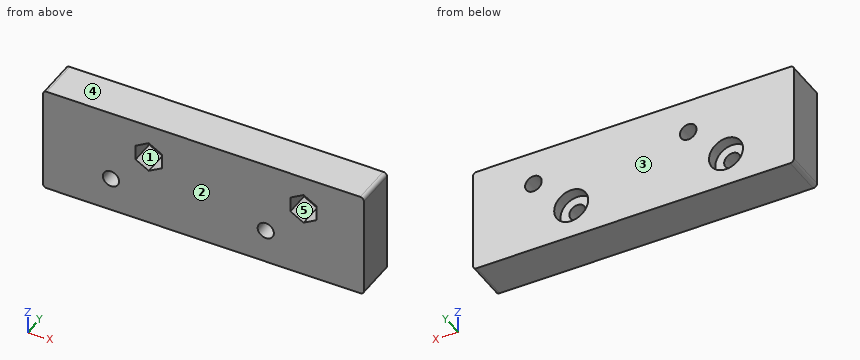
Autodesk Inventor part; units mm, degrees
ref_plane "YZ Plane" through (0, 0, 0) normal (1, 0, 0) x (0, 1, 0)
ref_plane "XZ Plane" through (0, 0, 0) normal (0, 1, 0) x (-1, 0, 0)
ref_plane "XY Plane" through (0, 0, 0) normal (0, 0, 1) x (1, 0, 0)
sketch "Esboço1" plane through (0, 0, 0) normal (0, 1, 0) x (-1, 0, 0)
  line L0 (0, 0) -> (77, 0)
  line L1 (77, 0) -> (77, -140)
  line L2 (77, -140) -> (0, -140)
  line L3 (0, -140) -> (0, 0)
  circle A0 centre (67, -20) radius 2.15
  circle A1 centre (67, -120) radius 2.15
  circle A2 centre (26, -20) radius 2.15
  circle A3 centre (26, -120) radius 2.15
  dimension "d0" = 77
  dimension "d1" = 140
  dimension "d2" = 4.3
  dimension "d3" = 4.3
  dimension "d4" = 4.3
  dimension "d5" = 4.3
  dimension "d6" = 10
  dimension "d7" = 10
  dimension "d8" = 20
  dimension "d9" = 20
  dimension "d10" = 20
  dimension "d11" = 20
  dimension "d12" = 26
  dimension "d13" = 26
extrude "Extrusão1" add sketch "Esboço1" along normal blind 11
sketch "Esboço2" plane through (0, 11, 0) normal (0, 1, 0) x (1, 0, 0)
  circle A0 centre (-67, 20) radius 2.15
  circle A1 centre (-26, 20) radius 2.15
  circle A2 centre (-26, 120) radius 2.15
  circle A3 centre (-67, 120) radius 2.15
  circle A4 centre (-67, 20) radius 4.5
  circle A5 centre (-67, 120) radius 2.15
  circle A6 centre (-67, 120) radius 4.5
  circle A7 centre (-26, 120) radius 2.15
  circle A8 centre (-26, 120) radius 4.5
  circle A9 centre (-26, 20) radius 2.15
  circle A10 centre (-26, 20) radius 4.5
  point P0 (0, 0)
  dimension "d16" = 9
  dimension "d17" = 9
  dimension "d18" = 9
  dimension "d19" = 9
extrude "Extrusão2" cut sketch "Esboço2" against normal blind 3 contours A3 | A4 | A6 | A8 | A10
sketch "Esboço3" plane through (0, 11, 0) normal (0, 1, 0) x (1, 0, 0)
  point P0 (0, 0)
sketch "Esboço4" plane through (0, 11, 0) normal (0, 1, 0) x (1, 0, 0)
  circle A0 centre (-57, 30) radius 2.2
  circle A1 centre (-57, 110) radius 2.2
  circle A2 centre (-67, 20) radius 2.15
  circle A3 centre (-67, 120) radius 2.15
  circle A4 centre (-16, 30) radius 2.2
  circle A5 centre (-16, 110) radius 2.2
  circle A6 centre (-26, 20) radius 2.15
  circle A7 centre (-26, 120) radius 2.15
  point P0 (0, 0)
  dimension "d22" = 4.4
  dimension "d23" = 4.4
  dimension "d24" = 10
  dimension "d25" = 10
  dimension "d26" = 10
  dimension "d27" = 10
  dimension "d28" = 4.4
  dimension "d29" = 4.4
  dimension "d30" = 10
  dimension "d31" = 10
  dimension "d32" = 10
  dimension "d33" = 10
extrude "Extrusão3" cut sketch "Esboço4" against normal blind 12 contours A0 | A1 | A4 | A5
sketch "Esboço5" plane through (0, 0, 0) normal (0, -1, 0) x (1, 0, 0)
  circle A0 centre (-57, -110) radius 2.2
  circle A1 centre (-16, -110) radius 2.2
  circle A2 centre (-16, -30) radius 2.2
  circle A3 centre (-57, -30) radius 2.2
  line L0 (-53.525, -112.0063) -> (-57, -114.0126)
  line L1 (-57, -114.0126) -> (-60.475, -112.0063)
  line L2 (-60.475, -112.0063) -> (-60.475, -107.9937)
  line L3 (-60.475, -107.9937) -> (-57, -105.9874)
  line L4 (-57, -105.9874) -> (-53.525, -107.9937)
  line L5 (-53.525, -107.9937) -> (-53.525, -112.0063)
  line L6 (-53.525, -32.0063) -> (-57, -34.0126)
  line L7 (-57, -34.0126) -> (-60.475, -32.0063)
  line L8 (-60.475, -32.0063) -> (-60.475, -27.9937)
  line L9 (-60.475, -27.9937) -> (-57, -25.9874)
  line L10 (-57, -25.9874) -> (-53.525, -27.9937)
  line L11 (-53.525, -27.9937) -> (-53.525, -32.0063)
  line L12 (-16, -105.9874) -> (-12.525, -107.9937)
  line L13 (-12.525, -107.9937) -> (-12.525, -112.0063)
  line L14 (-12.525, -112.0063) -> (-16, -114.0126)
  line L15 (-16, -114.0126) -> (-19.475, -112.0063)
  line L16 (-19.475, -112.0063) -> (-19.475, -107.9937)
  line L17 (-19.475, -107.9937) -> (-16, -105.9874)
  circle A4 centre (-16, -30) radius 2.2
  line L18 (-12.525, -32.0063) -> (-16, -34.0126)
  line L19 (-16, -34.0126) -> (-19.475, -32.0063)
  line L20 (-19.475, -32.0063) -> (-19.475, -27.9937)
  line L21 (-19.475, -27.9937) -> (-16, -25.9874)
  line L22 (-16, -25.9874) -> (-12.525, -27.9937)
  line L23 (-12.525, -27.9937) -> (-12.525, -32.0063)
  line L24 (-77, -140) -> (-77, 0)
  line L25 (0, 0) -> (0, -140)
  dimension "d36" = 6.95
  dimension "d37" = 6.95
  dimension "d38" = 6.95
  dimension "d39" = 6.95
extrude "Extrusão4" cut sketch "Esboço5" against normal blind 6.5 contours A0 | L0 L1 L2 L3 L4 L5 | L6 L7 L8 L9 L10 L11 | L12 L13 L14 L15 L16 L17 | L18 L19 L20 L21 L22 L23
sketch "Esboço6" plane through (-77, 0, 0) normal (0, 0, 1) x (1, 0, 0)
  line L0 (0, 0) -> (77, 0)
  line L1 (77, 0) -> (77, 11)
  line L2 (0, 11) -> (77, 11)
  line L3 (0, 0) -> (0, 11)
extrude "Extrusão5" add sketch "Esboço6" along normal blind 0.5
sketch "Esboço7" plane through (0, 0, -140) normal (0, 0, -1) x (-1, 0, 0)
  line L0 (0, 0) -> (77, 0)
  line L1 (77, 0) -> (77, 11)
  line L2 (0, 11) -> (77, 11)
  line L3 (0, 0) -> (0, 11)
  point P0 (0, 0)
extrude "Extrusão6" add sketch "Esboço7" along normal blind 0.5
sketch "Esboço8" plane through (-77, 0, 0.5) normal (-1, 0, 0) x (0, 0, 1)
  line L0 (0, 0) -> (-141, 0)
  line L1 (0, 11) -> (0, 0)
  line L2 (0, 11) -> (-141, 11)
  line L3 (-141, 0) -> (-141, 11)
  point P0 (-0.5, 0)
extrude "Extrusão7" add sketch "Esboço8" along normal blind 8
fillet "Arredondamento1" radius 1 4 edges at (-85, 5.5, 0.5) (0, 5.5, 0.5) (-85, 5.5, -140.5) (0, 5.5, -140.5)
sketch "Esboço9" plane through (0, 11, 0) normal (0, 1, 0) x (1, 0, 0)
  line L0 (0, 0.5) -> (0, 139.5)
  line L1 (-85, 139.5) -> (-85, 0.5)
  line L2 (0, 129) -> (-85, 129)
  line L3 (-85, 129) -> (-85, 101)
  line L4 (-85, 101) -> (0, 101)
  line L5 (0, 101) -> (0, 129)
  circle A0 centre (-16, 110) radius 2.2
  circle A1 centre (-26, 120) radius 4.5
  point P0 (0, 0)
  point P1 (0, 101)
  dimension "d49" = 9
  dimension "d50" = 9
extrude "Extrusão8" cut sketch "Esboço9" against normal mid plane 22 contours L4 L1 L2 L0 | A1 keep common part
fillet "Arredondamento2" radius 1 4 edges at (0, 5.5, -101) (0, 5.5, -129) (-85, 5.5, -101) (-85, 5.5, -129)
equation "\"d4\" = d3"
equation "\"d5\" = d3"
equation "\"d7\" = d6"
equation "\"d9\" = d8"
equation "\"d10\" = d9"
equation "\"d11\" = d8"
equation "\"d16\" = d19"
equation "\"d22\" = d28"
equation "\"d23\" = d29"
equation "\"d26\" = d25"
equation "\"d27\" = d26"
equation "\"d29\" = d28"
equation "\"d30\" = d24"
equation "\"d33\" = d32"
equation "\"d36\" = d39"
equation "\"d37\" = d39"
equation "\"d38\" = d39"
properties part number "suporte-fonte2"
Geometry check sheet. Reference: the model listing, model coordinates, mm. Face numbers are marked on the shaded views. A direction names the side the tool comes from. Give positions to 0.01 mm unless a question says otherwise; leave off trailing zeros. Write each loop counter-clockwise with the first axis right and the second up, starting at its lowest first coordinate (ties: lowest second). Pieces come first, ordered by that corner, then holes.
1) Section check B-B, the plane z = -110. Record the boundary of the cut face in (x, y) (3 decimals).
2) Section check C-C, the plane y = 9.25. Record the boundary of the cut face in (x, z).
3) Gauge pin test, flat ends, axial feed: pin 1 (3.5 mm diameter, centred on x = -26, z = -120, fed in from +Y); pin 2 (3.5 mm diameter, centred on x = -57.5, z = -109, fed in from -Y); pin 3 (2.5 mm diameter, centred on x = -65.5, z = -118, fed in from +Y). Record the tip position at first contact, or that the pin passes through.
4) Material ranges on L1, parallel to X at y = 9.25, z = -110; L2, parallel to X at y = 2, z = -109.75 (3 decimals); L3, parallel to Z at x = -67, y = 3.5, recorded low to high.
5) Section check D-D, the plane y = 5.5. Record the boundary of the cut face in (x, z) (3 decimals), and give its area (3 significant figures).
6) Section check A-A, the plane x = -67. Record the boundary of the cut face in (y, z).
7) Release check for a two-part mould opening along Z. For the marked faces 3, 4 and 5 record: pulls with the +Z half, pulls with the -Z half, needs draft (parallel to the pull), parting line crosses it, or undercut.
8) Access from +Z, -Z, +X, -X, +Y, -Y to the whole of each face (thin tool, end or side, straight path). Record for the marked faces 1 and 2.
Computed:
1. outline: (-85, 0) - (-60.475, 0) - (-60.475, 6.5) - (-59.2, 6.5) - (-59.2, 11) - (-85, 11) - close; (-54.8, 6.5) - (-53.525, 6.5) - (-53.525, 0) - (-19.475, 0) - (-19.475, 6.5) - (-18.2, 6.5) - (-18.2, 11) - (-54.8, 11) - close; (-13.8, 6.5) - (-12.525, 6.5) - (-12.525, 0) - (0, 0) - (0, 11) - (-13.8, 11) - close
2. outline: (-85, -128) arc R1 ccw to (-84, -129) - (-1, -129) arc R1 ccw to (0, -128) - (0, -102) arc R1 ccw to (-1, -101) - (-84, -101) arc R1 ccw to (-85, -102) - close; hole circle Ø9 at (-67, -120); hole circle Ø4.4 at (-57, -110); hole circle Ø9 at (-26, -120); hole circle Ø4.4 at (-16, -110)
3. pin 1: passes through
3. pin 2: stops at y = 6.5
3. pin 3: stops at y = 8
4. L1: x = -85 to -59.2, -54.8 to -18.2, -13.8 to 0
4. L2: x = -85 to -60.475, -53.525 to -19.475, -12.525 to 0
4. L3: z = -129 to -122.15, -117.85 to -101
5. outline: (-85, -128) arc R1 ccw to (-84, -129) - (-1, -129) arc R1 ccw to (0, -128) - (0, -102) arc R1 ccw to (-1, -101) - (-84, -101) arc R1 ccw to (-85, -102) - close; hole circle Ø4.3 at (-67, -120); hole (-60.475, -112.006) - (-57, -114.013) - (-53.525, -112.006) - (-53.525, -107.994) - (-57, -105.987) - (-60.475, -107.994) - close; hole circle Ø4.3 at (-26, -120); hole (-19.475, -112.006) - (-16, -114.013) - (-12.525, -112.006) - (-12.525, -107.994) - (-16, -105.987) - (-19.475, -107.994) - close
5. area: 2,270 mm2
6. outline: (0, -129) - (11, -129) - (11, -124.5) - (8, -124.5) - (8, -122.15) - (0, -122.15) - close; (0, -117.85) - (8, -117.85) - (8, -115.5) - (11, -115.5) - (11, -101) - (0, -101) - close
7. face 3: needs draft
7. face 4: pulls with the +Z half
7. face 5: undercut
8. face 1: -Y
8. face 2: +Z, -Z, +X, -X, -Y
